Read the model definition and answer for the solid it produces. Units are mm, in the model's axes. A direction names the side the tool comes from. Give positions to 0.01 mm unless a question says otherwise; leave off trailing zeros. Write each loop counter-clockwise with the first axis right and the second up, starting at its lowest first coordinate (ties: lowest second). Pieces come first, ordered by that corner, then holes. Notation, with made-up numbers: (11.25, 6.25) -> (18.25, 6.25) arc R27 cw to (18.25, 28.25) -> close; hole circle Ø4 at (-10.5, 82.5). An arc over 180 degrees is marked (long way). Use a Markdown table: item, result.
from build123d import *

# Parameters (mm, degrees)
BOSS_EXTRUDE1_DEPTH              = 38.1
SKETCH2_R                        = 39.62
BOSS_EXTRUDE2_DEPTH              = 120.65
F_1_16_1_25_DIAMETER_HOLE1_D     = 31.75
F_1_16_1_25_DIAMETER_HOLE1_DEPTH = 71.94630657
F_1_16_1_25_DIAMETER_HOLE1_TIP   = 4.25369343
SKETCH4_R                        = 19.05
CUT_EXTRUDE1_DEPTH               = 238.253258987
FILLET1_R                        = 3.81
SKETCH6_R                        = 10.922
CUT_EXTRUDE2_DEPTH               = 214.644491855
FILLET2_R                        = 2.54
F_1_16_2_5_DIAMETER_HOLE1_D      = 63.5
F_1_16_2_5_DIAMETER_HOLE1_DEPTH  = 67.69261314
F_1_16_2_5_DIAMETER_HOLE1_TIP    = 8.50738686


with BuildPart() as part:
    # Sketch1 → Boss-Extrude1 (new body)
    with BuildSketch(Plane(origin=(0, 0, 0), x_dir=(0, 0, -1), z_dir=(1, 0, 0))):
        with BuildLine():
            Line((-85.1, 69.32), (-85.1, 0))
            ThreePointArc((-85.1, 0), (0, -85.1), (85.1, 0))
            Line((85.1, 0), (85.1, 69.32))
            ThreePointArc((85.1, 69.32), (0, 154.42), (-85.1, 69.32))
        make_face()
    extrude(amount=-BOSS_EXTRUDE1_DEPTH)

    # Sketch2 → Boss-Extrude2 (add)
    with BuildSketch(Plane.ZY.offset(38.1)):
        with Locations(Location((0, 0, 0), (0, 0, 180))):
            Circle(SKETCH2_R)
    extrude(amount=BOSS_EXTRUDE2_DEPTH)

    # 1/16 (1.25) Diameter Hole1
    with Locations(Plane(origin=(-158.75, 0, 0), x_dir=(0, 0, -1), z_dir=(-1, 0, 0))):
        with Locations((0, 0)):
            Hole(F_1_16_1_25_DIAMETER_HOLE1_D / 2, depth=F_1_16_1_25_DIAMETER_HOLE1_DEPTH)
            with Locations((0, 0, -(F_1_16_1_25_DIAMETER_HOLE1_DEPTH + F_1_16_1_25_DIAMETER_HOLE1_TIP / 2))):  # 150° drill point
                Cone(0, F_1_16_1_25_DIAMETER_HOLE1_D / 2, F_1_16_1_25_DIAMETER_HOLE1_TIP, mode=Mode.SUBTRACT)

    # Sketch4 → Cut-Extrude1 (cut, through all)
    with BuildSketch(Plane.ZY.offset(158.75)):
        Circle(SKETCH4_R)
    extrude(amount=-CUT_EXTRUDE1_DEPTH, mode=Mode.SUBTRACT)

    # Fillet1
    fillet1_edges = [part.edges().sort_by_distance(p)[0] for p in [
        (-38.1, 0, 39.62),
    ]]
    fillet(fillet1_edges, radius=FILLET1_R)

    # Sketch6 → Cut-Extrude2 (cut, through all)
    with BuildSketch(Plane.ZY.offset(38.1)):
        with Locations((0, 132.831)):
            Circle(SKETCH6_R)
        with Locations((63.5, 69.331)):
            Circle(SKETCH6_R)
        with Locations((-63.5, 69.331)):
            Circle(SKETCH6_R)
        with Locations((63.5, -0.011)):
            Circle(SKETCH6_R)
        with Locations((0, -63.511)):
            Circle(SKETCH6_R)
        with Locations((-63.5, -0.011)):
            Circle(SKETCH6_R)
    extrude(amount=-CUT_EXTRUDE2_DEPTH, mode=Mode.SUBTRACT)

    # Fillet2
    fillet2_edges = [part.edges().sort_by_distance(p)[0] for p in [
        (-38.1, -85.1, 0),
        (-38.1, 34.66, -85.1),
        (-38.1, 154.42, 0),
        (-38.1, 34.66, 85.1),
    ]]
    fillet(fillet2_edges, radius=FILLET2_R)

    # 1/16 (2.5) Diameter Hole1
    with Locations(Plane(origin=(-158.75, 0, 0), x_dir=(0, 0, -1), z_dir=(-1, 0, 0))):
        with Locations((0, 0)):
            Hole(F_1_16_2_5_DIAMETER_HOLE1_D / 2, depth=F_1_16_2_5_DIAMETER_HOLE1_DEPTH)
            with Locations((0, 0, -(F_1_16_2_5_DIAMETER_HOLE1_DEPTH + F_1_16_2_5_DIAMETER_HOLE1_TIP / 2))):  # 150° drill point
                Cone(0, F_1_16_2_5_DIAMETER_HOLE1_D / 2, F_1_16_2_5_DIAMETER_HOLE1_TIP, mode=Mode.SUBTRACT)


solid = part.part
Item 1: For a pull along Z with two mould halves and no side action, classify faces 1 (the face through (-18, 34, -85.1)), 2 (the face through (0, 36, 1)), 3 (the face through (-87.87, 12.08, 15.75)), 4 (the face through (-17.5, 154.4, -1.9)) as +Z half, -Z half, draft (parallel to the pull), parting line (faces both ways), or undercut.
Return value:
| item | result |
|---|---|
| face 1 | -Z half |
| face 2 | draft |
| face 3 | undercut |
| face 4 | parting line |
Item 2: A cutting plane is placed at B-B (x = -13.5). Give the vertices of the cut face in (y, z), then the cut area to 3 significant figures.
Return value:
| item | result |
|---|---|
| outline | (0, -85.1) -> (69.32, -85.1) arc R85.1 ccw to (69.32, 85.1) -> (0, 85.1) arc R85.1 ccw to start; hole circle Ø21.84 at (-63.51, 0); hole circle Ø38.1 at (0, 0); hole circle Ø21.84 at (-0.01, -63.5); hole circle Ø21.84 at (-0.01, 63.5); hole circle Ø21.84 at (69.33, -63.5); hole circle Ø21.84 at (69.33, 63.5); hole circle Ø21.84 at (132.83, 0) |
| area | 31,200 mm^2 |
Item 3: A cutting plane is placed at C-C (x = -122.5). Give the vertices of the cut face in (y, z).
Return value:
| item | result |
|---|---|
| outline | circle Ø79.24 at (0, 0); hole circle Ø63.5 at (0, 0) |
Item 4: A cutting plane is placed at A-A (z = 0). Give the vertices of the cut face in (x, y), then the cut area to 3 significant figures.
Return value:
| item | result |
|---|---|
| outline | (-158.75, -39.62) -> (-41.91, -39.62) arc R3.81 cw to (-38.1, -43.43) -> (-38.1, -52.59) -> (0, -52.59) -> (0, -19.05) -> (-87.65, -19.05) -> (-91.06, -31.75) -> (-158.75, -31.75) -> close; (-158.75, 31.75) -> (-91.06, 31.75) -> (-87.65, 19.05) -> (0, 19.05) -> (0, 121.91) -> (-38.1, 121.91) -> (-38.1, 43.43) arc R3.81 cw to (-41.91, 39.62) -> (-158.75, 39.62) -> close; (-38.1, -82.56) arc R2.54 ccw to (-35.56, -85.1) -> (0, -85.1) -> (0, -74.43) -> (-38.1, -74.43) -> close; (-38.1, 143.75) -> (0, 143.75) -> (0, 154.42) -> (-35.56, 154.42) arc R2.54 ccw to (-38.1, 151.88) -> close |
| area | 9,210 mm^2 |
Item 5: Each of these flat-tipped pins is pushed along its axis until it touches: P1, Ø2, axis at x = -19, y = 99, coming from the -Z side; P2, Ø3, axis at y = 117.5, z = -14.5, coming from the -X side; P3, Ø6, axis at x = -35, y = -6.5, coming from the -Z side. Where does it stop, or does it pass through?
Return value:
| item | result |
|---|---|
| P1 | z = -80.12 |
| P2 | x = -38.1 |
| P3 | z = -85.03 |
Item 6: A tool of negligible diameter and unlimited length cuts with its end or side. For faces 5 (the face through (-38.1, 62, 1)), 6 (the face through (-19.32, 143.66, -1.42)), from which of +Z, -Z, +X, -X, +Y, -Y can it reach the whole face along a straight path? Write none if from no direction.
Return value:
| item | result |
|---|---|
| face 5 | -X |
| face 6 | +X, -X |
Item 7: A cutting plane is placed at D-D (z = 68). Count the separate pieces of the cut face and the enclosed holes in it, then the cut area to 3 significant figures.
Return value:
| item | result |
|---|---|
| separate pieces | 3 |
| enclosed holes | 0 |
| area | 5,020 mm^2 |
Item 8: Straight lines are drawn through the part: line 1 along Y through (x, z) = (-27, 0); line 2 along Y through (x, z) = (-74, 1.5); line 3 along Y through (x, z) = (-130.5, 0). For each, find the intervals that lie inside material, in ascending order. Write a range as [from, to].
Return value:
| item | result |
|---|---|
| line 1 | [-85.1, -74.43], [-52.59, -19.05], [19.05, 121.91], [143.75, 154.42] |
| line 2 | [-39.59, -18.99], [18.99, 39.59] |
| line 3 | [-39.62, -31.75], [31.75, 39.62] |
